Geometry: final body of the model. Coordinates: model frame, mm. Face numbers are marked on the shaded views. A direction names the side the tool comes from. Round coordinates to 2 decimals unless told otherwise and drop trailing zeros. Order: outer loops, then holes, each group sorted by start corner. A loop starts at its lowest first (then second) coordinate and runs counter-clockwise, first axis right, second up. Notation, with made-up numbers: M 36,-38.5 L 72,-38.5 A22 cw 72,0.5 Z; hole C 18.25,35.25 d3. An arc over 180 degrees is marked long. Put each result on its own line as item: value. Start each with the question number.
1) Access query for the marked faces 1, 2 and 3. Directions: +Z, -Z, +X, -X, +Y, -Y. A direction counts if a zero-diameter tool reaches every point of the face in a straight line with its end or side. Return the directions, or none.
2) Material intervals for probe 1 along X at (y, z) = (19.75, -10.75) (3 decimals); probe 2 along Y at (x, z) = (61.25, -12.7); probe 3 along X at (y, z) = (9.75, -13.5), sorted ascending. Write a range as [from, to].
3) Section A-A, the plane z = -12.7. Count the separate pieces of the cut face and the enclosed holes in it, then the cut area to 3 significant figures.
4) First-contact query: P1, Ø7.5, axis at y = 14, z = -11.5, coming from the -X side; P2, Ø12, axis at y = 16.5, z = -14, coming from the -X side; P3, Ø0.6, axis at x = 58.5, z = -11.5, coming from the +Y side. Flat tips, straight axial feed; report the tip coordinate or a pass-through.
5) Section B-B, the plane x = 73.5. Return loops of the section in (y, z).
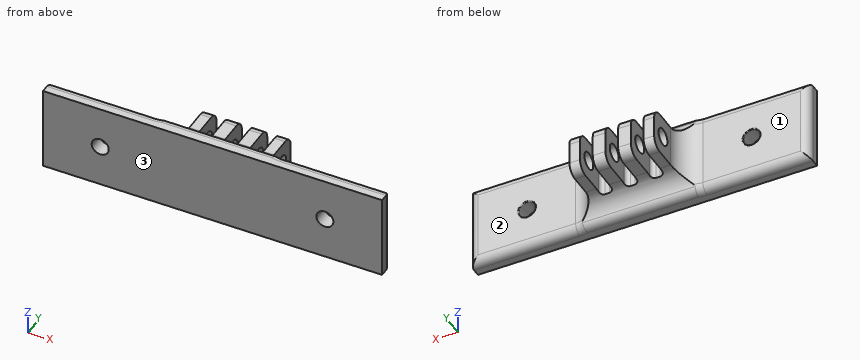
from build123d import *
from build123d.topology import SkipClean

# Parameters (mm, degrees)
SKETCH1_W           = 101.6
SKETCH1_H           = 25.4
BOSS_EXTRUDE1_DEPTH = 4.7625
SKETCH2_W           = 25.4
SKETCH2_H           = 12.7
BOSS_EXTRUDE2_DEPTH = 15.875
SKETCH3_W           = 3.81
SKETCH3_H           = 12.065
CUT_EXTRUDE1_DEPTH  = 25.4
SKETCH4_R           = 2.5781
CUT_EXTRUDE2_DEPTH  = 72.4375
FILLET2_START       = 45.085
FILLET2_DEPTH       = 3.81
FILLET2_START_2     = 52.705
FILLET2_2_DEPTH     = 3.81
FILLET2_START_3     = 38.1
FILLET2_3_DEPTH     = 3.175
FILLET2_START_4     = 60.325
FILLET2_4_DEPTH     = 3.175
FILLET2_START_5     = -25.4
FILLET2_5_OUTLINE_W = 3.81
FILLET2_5_OUTLINE_H = 3.81
FILLET2_5_DEPTH     = 25.4
FILLET2_6_DEPTH     = 101.6
FILLET3_2_DEPTH     = 101.6
FILLET3_3_DEPTH     = 31.75
FILLET3_START       = 69.85
FILLET3_4_DEPTH     = 31.75
FILLET3_START_2     = -26
FILLET3_5_DEPTH     = 27
FILLET4_R           = 3.175
FILLET5_R           = 1.27
SKETCH5_R           = 2.5527
CUT_EXTRUDE3_DEPTH  = 106.923253491
FILLET6_R           = 0.254


with BuildPart() as part:
    # Sketch1 → Boss-Extrude1 (new body)
    with BuildSketch(Plane(origin=(0, 0, 0), x_dir=(1, 0, 0), z_dir=(0, 1, 0))):
        with Locations((50.8, 12.7)):
            Rectangle(SKETCH1_W, SKETCH1_H)
    extrude(amount=BOSS_EXTRUDE1_DEPTH)

    # Sketch2 → Boss-Extrude2 (add)
    with BuildSketch(Plane(origin=(0, 4.7625, 0), x_dir=(1, 0, 0), z_dir=(0, 1, 0))):
        with Locations((50.8, 12.7)):
            Rectangle(SKETCH2_W, SKETCH2_H)
    extrude(amount=BOSS_EXTRUDE2_DEPTH)

    # Sketch3 → Cut-Extrude1 (cut)
    with BuildSketch(Plane.XY.offset(-6.35)):
        with Locations((50.8, 14.605)):
            Rectangle(SKETCH3_W, SKETCH3_H)
        with Locations((43.18, 14.605)):
            Rectangle(SKETCH3_W, SKETCH3_H)
        with Locations((58.42, 14.605)):
            Rectangle(SKETCH3_W, SKETCH3_H)
    extrude(amount=-CUT_EXTRUDE1_DEPTH, mode=Mode.SUBTRACT)

    # Sketch4 → Cut-Extrude2 (cut, through all)
    with BuildSketch(Plane(origin=(63.5, 0, 0), x_dir=(0, 0, -1), z_dir=(1, 0, 0))):
        with Locations((12.7, 15.5575)):
            Circle(SKETCH4_R)
    extrude(amount=-CUT_EXTRUDE2_DEPTH, mode=Mode.SUBTRACT)

    # Fillet2: read off the stored shape, not the designer's step
    # Fillet2 outline → Fillet2 (add)
    with BuildSketch(Plane.YZ.offset(FILLET2_START)):
        with BuildLine():
            Line((4.7625, -6.35), (11.1125, -6.35))
            ThreePointArc((11.1125, -6.35), (6.622371939, -4.490128061), (4.7625, 0))
            Line((4.7625, 0), (4.7625, -6.35))
        make_face()
        with BuildLine():
            Line((11.1125, -19.05), (4.7625, -19.05))
            Line((4.7625, -19.05), (4.7625, -25.4))
            ThreePointArc((4.7625, -25.4), (6.622371939, -20.909871939), (11.1125, -19.05))
        make_face()
    extrude(amount=FILLET2_DEPTH)

    # Fillet2 2 outline → Fillet2 2 (add)
    with BuildSketch(Plane.YZ.offset(FILLET2_START_2)):
        with BuildLine():
            Line((4.7625, -6.35), (11.1125, -6.35))
            ThreePointArc((11.1125, -6.35), (6.622371939, -4.490128061), (4.7625, 0))
            Line((4.7625, 0), (4.7625, -6.35))
        make_face()
        with BuildLine():
            Line((11.1125, -19.05), (4.7625, -19.05))
            Line((4.7625, -19.05), (4.7625, -25.4))
            ThreePointArc((4.7625, -25.4), (6.622371939, -20.909871939), (11.1125, -19.05))
        make_face()
    extrude(amount=FILLET2_2_DEPTH)

    # Fillet2 3 outline → Fillet2 3 (add)
    with BuildSketch(Plane.YZ.offset(FILLET2_START_3)):
        with BuildLine():
            Line((4.7625, -6.35), (11.1125, -6.35))
            ThreePointArc((11.1125, -6.35), (6.622371939, -4.490128061), (4.7625, 0))
            Line((4.7625, 0), (4.7625, -6.35))
        make_face()
        with BuildLine():
            Line((11.1125, -19.05), (4.7625, -19.05))
            Line((4.7625, -19.05), (4.7625, -25.4))
            ThreePointArc((4.7625, -25.4), (6.622371939, -20.909871939), (11.1125, -19.05))
        make_face()
    extrude(amount=FILLET2_3_DEPTH)

    # Fillet2 4 outline → Fillet2 4 (add)
    with BuildSketch(Plane.YZ.offset(FILLET2_START_4)):
        with BuildLine():
            Line((4.7625, -6.35), (11.1125, -6.35))
            ThreePointArc((11.1125, -6.35), (6.622371939, -4.490128061), (4.7625, 0))
            Line((4.7625, 0), (4.7625, -6.35))
        make_face()
        with BuildLine():
            Line((11.1125, -19.05), (4.7625, -19.05))
            Line((4.7625, -19.05), (4.7625, -25.4))
            ThreePointArc((4.7625, -25.4), (6.622371939, -20.909871939), (11.1125, -19.05))
        make_face()
    extrude(amount=FILLET2_4_DEPTH)

    # Fillet2 5 outline → Fillet2 5 (add)
    with BuildSketch(Plane.XY.offset(FILLET2_START_5)):
        with BuildLine():
            ThreePointArc((69.85, 4.7625), (65.359871939, 6.622371939), (63.5, 11.1125))
            Line((63.5, 11.1125), (63.5, 4.7625))
            Line((63.5, 4.7625), (69.85, 4.7625))
        make_face()
        with BuildLine():
            Line((38.1, 4.7625), (38.1, 11.1125))
            ThreePointArc((38.1, 11.1125), (36.240128061, 6.622371939), (31.75, 4.7625))
            Line((31.75, 4.7625), (38.1, 4.7625))
        make_face()
        with Locations((58.42, 6.6675)):
            Rectangle(FILLET2_5_OUTLINE_W, FILLET2_5_OUTLINE_H)
        with Locations((43.18, 6.6675)):
            Rectangle(FILLET2_5_OUTLINE_W, FILLET2_5_OUTLINE_H)
        with Locations((50.8, 6.6675)):
            Rectangle(FILLET2_5_OUTLINE_W, FILLET2_5_OUTLINE_H)
    extrude(amount=FILLET2_5_DEPTH)

    # Fillet2 6 outline → Fillet2 6 (cut)
    with SkipClean():  # the faces are left unmerged after this step: merging them gives an invalid solid
        with BuildSketch(Plane.YZ):
            with BuildLine():
                Line((11.1125, -6.35), (13, -6.35))
                Line((13, -6.35), (13, 0))
                Line((13, 0), (4.7625, 0))
                ThreePointArc((4.7625, 0), (6.622371939, -4.490128061), (11.1125, -6.35))
            make_face()
            with BuildLine():
                Line((4.7625, -25.4), (13, -25.4))
                Line((13, -25.4), (13, -19.05))
                Line((13, -19.05), (11.1125, -19.05))
                ThreePointArc((11.1125, -19.05), (6.622371939, -20.909871939), (4.7625, -25.4))
            make_face()
        extrude(amount=FILLET2_6_DEPTH, mode=Mode.SUBTRACT)
    add(part.part.scale(1), mode=Mode.REPLACE)  # the faces are merged on a copy

    # Fillet3: read off the stored shape, not the designer's step
    # Fillet3 outline → Fillet3 (revolve, cut)
    with BuildSketch(Plane(origin=(31.75, 11.1125, 0), x_dir=(1, 0, 0), z_dir=(0, -1, 0))):
        with BuildLine():
            Line((6.35, 0), (6.35, -2.54))
            ThreePointArc((6.35, -2.54), (7.093948776, -0.743948776), (8.89, 0))
            Line((8.89, 0), (6.35, 0))
        make_face()
        with BuildLine():
            ThreePointArc((8.89, -25.4), (7.093948776, -24.656051224), (6.35, -22.86))
            Line((6.35, -22.86), (6.35, -25.4))
            Line((6.35, -25.4), (8.89, -25.4))
        make_face()
    revolve(axis=Axis((31.75, 11.1125, 0), (0, 0, 1)), mode=Mode.SUBTRACT)

    # Fillet3 2 outline → Fillet3 2 (cut)
    with BuildSketch(Plane.YZ):
        with BuildLine():
            Line((4.7625, 0), (2.593081006, 0))
            ThreePointArc((2.593081006, 0), (4.111021339, -0.503469337), (5.027200718, -1.814285714))
            ThreePointArc((5.027200718, -1.814285714), (4.829023636, -0.916746847), (4.7625, 0))
        make_face()
        with BuildLine():
            Line((2.593081006, -25.4), (4.7625, -25.4))
            ThreePointArc((4.7625, -25.4), (4.829023636, -24.483253153), (5.027200718, -23.585714286))
            ThreePointArc((5.027200718, -23.585714286), (4.111021339, -24.896530663), (2.593081006, -25.4))
        make_face()
    extrude(amount=FILLET3_2_DEPTH, mode=Mode.SUBTRACT)

    # Fillet3 3 outline → Fillet3 3 (cut)
    with BuildSketch(Plane.YZ):
        with BuildLine():
            ThreePointArc((4.7625, -1.218931786), (3.837284915, -0.325602422), (2.593081006, 0))
            Line((2.593081006, 0), (2.2225, 0))
            ThreePointArc((2.2225, 0), (4.018551224, -0.743948776), (4.7625, -2.54))
            Line((4.7625, -2.54), (4.7625, -1.218931786))
        make_face()
        with BuildLine():
            Line((4.7625, -24.181068214), (4.7625, -22.86))
            ThreePointArc((4.7625, -22.86), (4.018551224, -24.656051224), (2.2225, -25.4))
            Line((2.2225, -25.4), (2.593081006, -25.4))
            ThreePointArc((2.593081006, -25.4), (3.837284915, -25.074397578), (4.7625, -24.181068214))
        make_face()
    extrude(amount=FILLET3_3_DEPTH, mode=Mode.SUBTRACT)

    # Fillet3 4 outline → Fillet3 4 (cut)
    with BuildSketch(Plane.YZ.offset(FILLET3_START)):
        with BuildLine():
            ThreePointArc((4.7625, -1.218931786), (3.837284915, -0.325602422), (2.593081006, 0))
            Line((2.593081006, 0), (2.2225, 0))
            ThreePointArc((2.2225, 0), (4.018551224, -0.743948776), (4.7625, -2.54))
            Line((4.7625, -2.54), (4.7625, -1.218931786))
        make_face()
        with BuildLine():
            Line((4.7625, -24.181068214), (4.7625, -22.86))
            ThreePointArc((4.7625, -22.86), (4.018551224, -24.656051224), (2.2225, -25.4))
            Line((2.2225, -25.4), (2.593081006, -25.4))
            ThreePointArc((2.593081006, -25.4), (3.837284915, -25.074397578), (4.7625, -24.181068214))
        make_face()
    extrude(amount=FILLET3_4_DEPTH, mode=Mode.SUBTRACT)

    # Fillet3 5 outline → Fillet3 5 (cut)
    with BuildSketch(Plane.XY.offset(FILLET3_START_2)):
        with BuildLine():
            Line((101.6, 4.7625), (99.06, 4.7625))
            ThreePointArc((99.06, 4.7625), (100.856051224, 4.018551224), (101.6, 2.2225))
            Line((101.6, 2.2225), (101.6, 4.7625))
        make_face()
        with BuildLine():
            ThreePointArc((0, 2.2225), (0.743948776, 4.018551224), (2.54, 4.7625))
            Line((2.54, 4.7625), (0, 4.7625))
            Line((0, 4.7625), (0, 2.2225))
        make_face()
    extrude(amount=FILLET3_5_DEPTH, mode=Mode.SUBTRACT)

    # Fillet3 6 outline → Fillet3 6 (revolve, cut)
    with BuildSketch(Plane(origin=(69.85, 11.1125, 0), x_dir=(1, 0, 0), z_dir=(0, -1, 0))):
        with BuildLine():
            Line((6.35, 0), (6.35, -2.54))
            ThreePointArc((6.35, -2.54), (7.093948776, -0.743948776), (8.89, 0))
            Line((8.89, 0), (6.35, 0))
        make_face()
        with BuildLine():
            ThreePointArc((8.89, -25.4), (7.093948776, -24.656051224), (6.35, -22.86))
            Line((6.35, -22.86), (6.35, -25.4))
            Line((6.35, -25.4), (8.89, -25.4))
        make_face()
    revolve(axis=Axis((69.85, 11.1125, 0), (0, 0, 1)), mode=Mode.SUBTRACT)

    # Fillet4
    fillet4_edges = [part.edges().sort_by_distance(p)[0] for p in [
        (39.6875, 20.6375, -6.35),
        (61.9125, 20.6375, -19.05),
        (46.99, 20.6375, -6.35),
        (54.61, 20.6375, -6.35),
        (61.9125, 20.6375, -6.35),
        (54.61, 20.6375, -19.05),
        (46.99, 20.6375, -19.05),
        (39.6875, 20.6375, -19.05),
    ]]
    fillet(fillet4_edges, radius=FILLET4_R)

    # Fillet5
    fillet5_edges = [part.edges().sort_by_distance(p)[0] for p in [
        (60.325, 8.5725, -12.7),
        (56.515, 8.5725, -12.7),
        (45.085, 8.5725, -12.7),
        (41.275, 8.5725, -12.7),
        (52.705, 8.5725, -12.7),
        (48.895, 8.5725, -12.7),
    ]]
    fillet(fillet5_edges, radius=FILLET5_R)

    # Sketch5 → Cut-Extrude3 (cut, through all)
    with BuildSketch(Plane(origin=(0, 4.7625, 0), x_dir=(1, 0, 0), z_dir=(0, 1, 0))):
        with Locations(Location((17.145, 12.7, 0), (0, 0, 270))):
            Circle(SKETCH5_R)
        with Locations(Location((84.455, 12.7, 0), (0, 0, 270))):
            Circle(SKETCH5_R)
    extrude(amount=-CUT_EXTRUDE3_DEPTH, mode=Mode.SUBTRACT)

    # Fillet6
    fillet6_edges = [part.edges().sort_by_distance(p)[0] for p in [
        (17.145, 4.7625, -15.2527),
        (84.455, 4.7625, -15.2527),
    ]]
    fillet(fillet6_edges, radius=FILLET6_R)


solid = part.part
Result sheet:
1. face 1: +Z, -Z, -X, +Y
1. face 2: +Z, -Z, +X, +Y
1. face 3: +Z, -Z, +X, -X, -Y
2. probe 1: x = [38.1, 41.275], [45.085, 48.895], [52.705, 56.515], [60.325, 63.5]
2. probe 2: y = [0, 12.98], [18.14, 20.64]
2. probe 3: x = [37.95, 41.28], [45.08, 48.9], [52.7, 56.52], [60.32, 63.65]
3. separate pieces: 7
3. enclosed holes: 0
3. area: 645 mm2
4. P1: stops at x = 38.04
4. P2: stops at x = 38.07
4. P3: stops at y = 8.57
5. outline: M 0,-25.4 L 2.22,-25.4 A2.54 ccw 4.76,-22.86 L 4.76,-2.54 A2.54 ccw 2.22,0 L 0,0 Z
